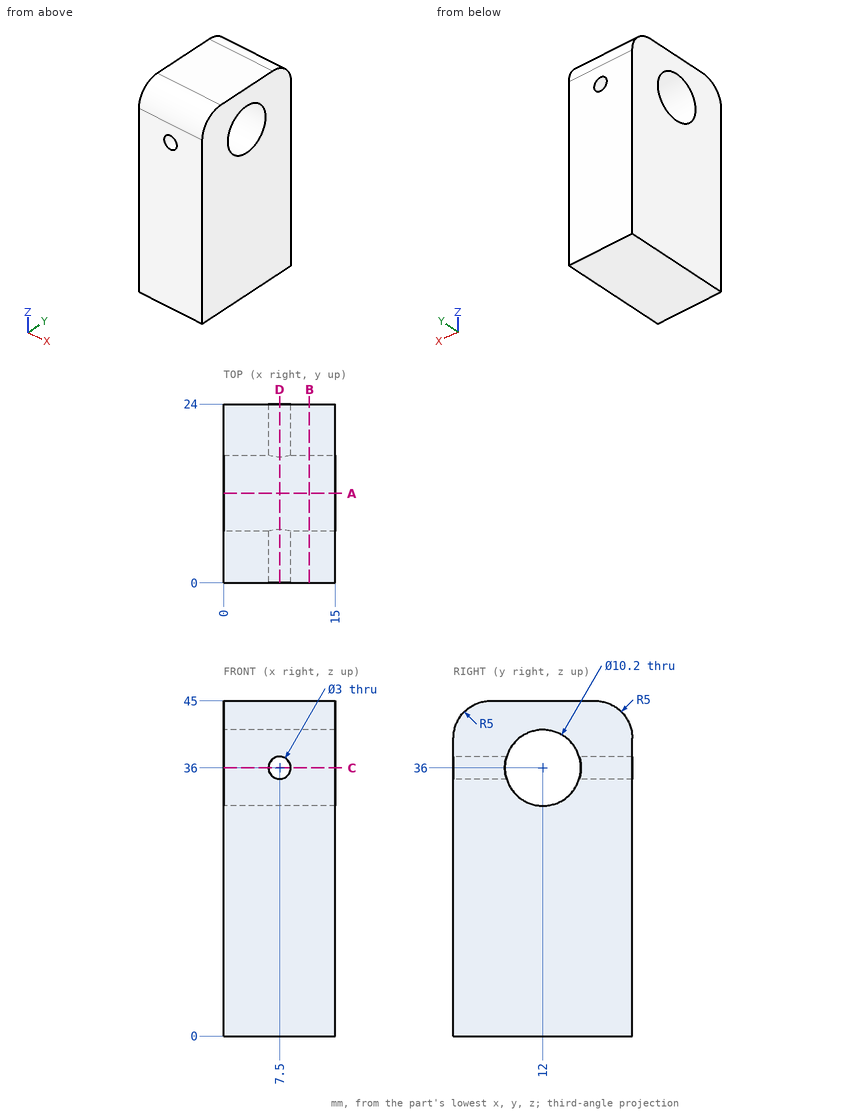
Could you check a few things on this drawing? It's one solid part, dimensions in mm from its lowest x, y, z. Round coordinates to 2 decimals unless told otherwise and drop trailing zeros. Loops run counter-clockwise (first coordinate to the right, second up) from the corner with the lowest first, then second, coordinate; pieces in that order, holes last. Notation, with made-up numbers: M 60,31.5 L 77,31.5 A12 cw 77,47.5 Z; hole C 80,-23 d2. An arc over 180 degrees is marked long. Write each question's results on one line, items separated by ' | '. Start each with the question number.
(1) If I drill on probe 1 along Y at (x, z) = (10.25, 36); probe 2 along Z at (x, y) = (7.5, 4.75); probe 3 along Z at (x, y) = (13.25, 12.75), over which ranges is the centre line in solid material (lowest first)? Write a range as from..to.
(2) I want a section at B-B (x = 11.5). Please give me the cut outline in (y, z).
(3) I want a section at C-C (z = 36). Please give me the cut outline in (x, y).
(4) I want a section at A-A (y = 12). Please give me the cut outline in (x, z), then the cut area to 3 significant figures.
(5) I want a section at D-D (x = 7.5). Please give me the cut outline in (y, z), then the cut area to 3 significant figures.
Solved:
1) probe 1: y = 0..6.9, 17.1..24 | probe 2: z = 0..34.5, 37.5..44.99 | probe 3: z = 0..30.96, 41.04..45
2) outline: M 0,0 L 24,0 L 24,40 A5 ccw 19,45 L 5,45 A5 ccw 0,40 Z; hole C 12,36 d10.2
3) outline: M 0,0 L 6,0 L 6,6.9 L 0,6.9 Z; M 0,17.1 L 6,17.1 L 6,24 L 0,24 Z; M 9,0 L 15,0 L 15,6.9 L 9,6.9 Z; M 9,17.1 L 15,17.1 L 15,24 L 9,24 Z
4) outline: M 0,0 L 15,0 L 15,30.9 L 0,30.9 Z; M 0,41.1 L 15,41.1 L 15,45 L 0,45 Z | area: 522 mm²
5) outline: M 0,0 L 24,0 L 24,34.5 L 16.87,34.5 A5.1 cw 7.13,34.5 L 0,34.5 Z; M 0,37.5 L 7.13,37.5 A5.1 cw 16.87,37.5 L 24,37.5 L 24,40 A5 ccw 19,45 L 5,45 A5 ccw 0,40 Z | area: 946 mm²
